Can you work these out from the model? Positions are in its coordinate system, mm. Face numbers are marked on the shaded views. Give positions to 0.01 mm unless a question says otherwise; leave off trailing zeros. Answer as a JSON object with one key per item and string values.
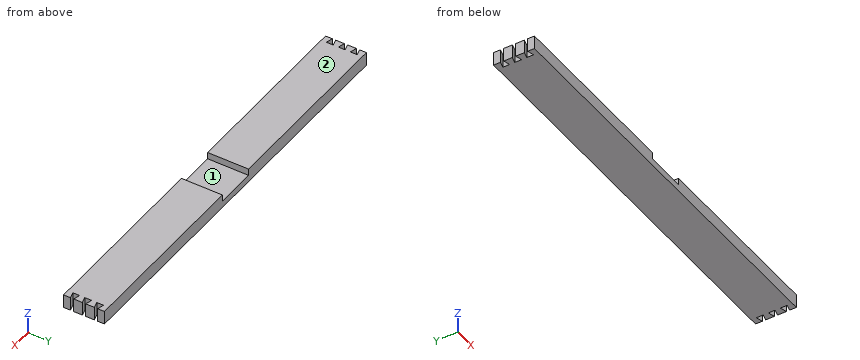
```python
from build123d import *

# Parameters (mm, degrees)
F1_DEPTH = 38.1
F3_DEPTH = 25.401


with BuildPart() as f1:
    # F0 (on Front) → F1 (new body, symmetric)
    with BuildSketch(Plane.XZ):
        Polygon((-38.1, 12.7), (-381, 12.7), (-381, -12.7), (381, -12.7), (381, 12.7), (38.1, 12.7), (38.1, 0), (-38.1, 0), align=None)
    extrude(amount=F1_DEPTH, both=True)

    # F2 (on face) → F3 (cut, through all)
    with BuildSketch(Plane.XY.offset(12.7)):
        Polygon((-368.732742, 15.987002), (-368.732742, 28.687002), (-381, 25.4), (-381, 19.274004), align=None)
        Polygon((-368.732742, 6.35), (-381, 3.062998), (-381, -3.062998), (-368.732742, -6.35), align=None)
        Polygon((-368.732742, -28.687002), (-368.732742, -15.987002), (-381, -19.274004), (-381, -25.4), align=None)
        Polygon((381, 19.274004), (381, 25.4), (368.732742, 28.687002), (368.732742, 15.987002), align=None)
        Polygon((381, -3.062998), (381, 3.062998), (368.732742, 6.35), (368.732742, -6.35), align=None)
        Polygon((381, -25.4), (381, -19.274004), (368.732742, -15.987002), (368.732742, -28.687002), align=None)
    extrude(amount=-F3_DEPTH, mode=Mode.SUBTRACT)


solid = f1.part
```
1) If we mould it in two halves opening along X, with no side actions, what happens to the marked faces 1 and 2? For each: released by +X, released by -X, zero draft, split by the parting line, or undercut.
Check sheet entries:
{"face 1": "undercut", "face 2": "zero draft"}
2) I need wall thicknesses on L1, parallel to X at y = 20, z = 7.75; L2, parallel to X at y = -7, z = 10; L3, parallel to Z at x = 5.5, y = -12. Which ranges of each line are inside material? Lowest first, please.
Check sheet entries:
{"L1": "-368.73 to -38.1, 38.1 to 368.73", "L2": "-381 to -38.1, 38.1 to 381", "L3": "-12.7 to 0"}
3) I'm going to push a flat-ended pin straight in: P1, Ø8, axis at y = 0.5, z = -5, coming from the +X side. Where does the tip first touch, or does it pass through?
Check sheet entries:
{"P1": "x = 381"}
